from build123d import *

# Parameters (mm, degrees)
SKETCH2_W     = 6.985
SKETCH2_H     = 32.356336156
SKETCH2_W_2   = 40.972237954
SKETCH2_H_2   = 0.889
CUTOUT_DEPTH  = 10.16
TAB_DEPTH     = 2.54
TAB_CHMF_SIZE = 1.524
CROSS_DEPTH   = 7.62
SKETCH4_W     = 3.302
SKETCH4_H     = 7.6962
BOX_DEPTH     = 13.059399
SKETCH6_W     = 1.778
SKETCH6_H     = 6.1722
BOXCUT_DEPTH  = 13.059399
FILLET1_R     = 1.27


with BuildPart() as part:
    # Sketch1 → dome/base (revolve)
    with BuildSketch(Plane.XY):
        with BuildLine():
            Line((0, 6.039891065), (0, 3.960890157))
            Line((0, 3.960890157), (8.222, 3.960890157))
            Line((8.222, 3.960890157), (8.222, -9.047708935))
            Line((8.222, -9.047708935), (10, -9.047708935))
            Line((10, -9.047708935), (10, 4.421422334))
            ThreePointArc((10, 4.421422334), (9.66312833, 5.282916106), (8.831225953, 5.687381775))
            ThreePointArc((8.831225953, 5.687381775), (4.419129287, 5.951728667), (0, 6.039891065))
        make_face()
    revolve(axis=Axis((0, 0, 0), (0, 1, 0)))

    # Sketch2 → cutout (cut)
    with BuildSketch(Plane.XZ.offset(9.047708935)):
        Rectangle(SKETCH2_W, SKETCH2_H)
        with Locations((0, 2.54)):
            Rectangle(SKETCH2_W_2, SKETCH2_H_2)
        with Locations((0, -2.54)):
            Rectangle(SKETCH2_W_2, SKETCH2_H_2)
    extrude(amount=-CUTOUT_DEPTH, mode=Mode.SUBTRACT)

    # Sketch3 → tab (add)
    with BuildSketch(Plane.XZ.offset(9.047708935)):
        with BuildLine():
            Line((-13.169324385, -2.0955), (-9.777979329, -2.0955))
            ThreePointArc((-9.777979329, -2.0955), (-10, 0), (-9.777979329, 2.0955))
            Line((-9.777979329, 2.0955), (-13.169324385, 2.0955))
            ThreePointArc((-13.169324385, 2.0955), (-13.335, 0), (-13.169324385, -2.0955))
        make_face()
        with BuildLine():
            Line((9.777979329, -2.0955), (13.169324385, -2.0955))
            ThreePointArc((13.169324385, -2.0955), (13.293516571, -1.051019583), (13.335, 0))
            ThreePointArc((13.335, 0), (13.293516571, 1.051019583), (13.169324385, 2.0955))
            Line((13.169324385, 2.0955), (9.777979329, 2.0955))
            ThreePointArc((9.777979329, 2.0955), (10, 0), (9.777979329, -2.0955))
        make_face()
    extrude(amount=-TAB_DEPTH)

    # tab chmf
    tab_chmf_edges = [part.edges().sort_by_distance(p)[0] for p in [
        (-13.335, -9.047708935, 0),
        (13.335, -9.047708935, 0),
    ]]
    chamfer(tab_chmf_edges, length=TAB_CHMF_SIZE)

    # Sketch5 → cross (add)
    with BuildSketch(Plane.XZ.offset(-3.960890157)):
        with BuildLine():
            Line((0, -0.71842049), (-0.71842049, 0))
            Line((-0.71842049, 0), (-6.161934605, -5.443514115))
            ThreePointArc((-6.161934605, -5.443514115), (-5.813831955, -5.813831955), (-5.443514115, -6.161934605))
            Line((-5.443514115, -6.161934605), (0, -0.71842049))
        make_face()
        with BuildLine():
            Line((6.161934605, -5.443514115), (0.71842049, 0))
            Line((0.71842049, 0), (0, -0.71842049))
            Line((0, -0.71842049), (5.443514115, -6.161934605))
            ThreePointArc((5.443514115, -6.161934605), (5.813831955, -5.813831955), (6.161934605, -5.443514115))
        make_face()
        with BuildLine():
            Line((5.443514115, 6.161934605), (0, 0.71842049))
            Line((0, 0.71842049), (0.71842049, 0))
            Line((0.71842049, 0), (6.161934605, 5.443514115))
            ThreePointArc((6.161934605, 5.443514115), (5.813831955, 5.813831955), (5.443514115, 6.161934605))
        make_face()
        Polygon((0.71842049, 0), (0, 0.71842049), (-0.71842049, 0), (0, -0.71842049), align=None)
        with BuildLine():
            Line((-0.71842049, 0), (0, 0.71842049))
            Line((0, 0.71842049), (-5.443514115, 6.161934605))
            ThreePointArc((-5.443514115, 6.161934605), (-5.813831955, 5.813831955), (-6.161934605, 5.443514115))
            Line((-6.161934605, 5.443514115), (-0.71842049, 0))
        make_face()
    extrude(amount=CROSS_DEPTH)

    # Sketch4 → box (add)
    with BuildSketch(Plane.XZ.offset(-3.960890157)):
        Rectangle(SKETCH4_W, SKETCH4_H)
    extrude(amount=BOX_DEPTH)

    # Sketch6 → boxcut (cut)
    with BuildSketch(Plane.XZ.offset(9.098508935)):
        Rectangle(SKETCH6_W, SKETCH6_H)
    extrude(amount=-BOXCUT_DEPTH, mode=Mode.SUBTRACT)

    # Fillet1
    fillet1_edges = [part.edges().sort_by_distance(p)[0] for p in [
        (-3.4925, -9.047708935, -8.406831929),
        (3.4925, -9.047708935, -8.406831929),
        (8.602728257, -9.047708935, -2.9845),
        (-8.602728257, -9.047708935, -2.9845),
        (-3.4925, -9.047708935, 8.406831929),
        (3.4925, -9.047708935, 8.406831929),
        (-8.602728257, -9.047708935, 2.9845),
        (8.602728257, -9.047708935, 2.9845),
    ]]
    fillet(fillet1_edges, radius=FILLET1_R)


solid = part.part
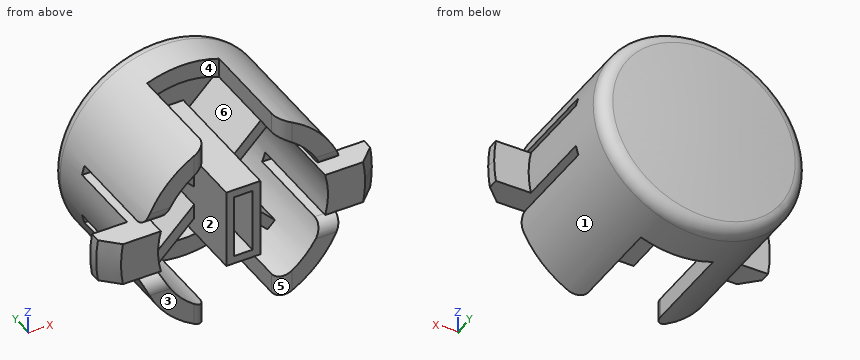
Design review of the part built by this model. Coordinates are the model's own, in mm. Face numbers are marked on the shaded views. A direction names the side the tool comes from. Round coordinates to 2 decimals unless told otherwise and drop trailing zeros. Loops run counter-clockwise (first coordinate to the right, second up) from the corner with the lowest first, then second, coordinate; pieces in that order, holes last. Notation, with made-up numbers: (20.25, 55) - (53.25, 55) arc R14 ccw to (53.25, 81) - close; hole circle Ø4 at (-3, 17.5). An arc over 180 degrees is marked (long way). One line per question, with ' | ' between items.
1. We need section C-C, the plane y = 5. State the section outline as (x, z) points.
Results are:
outline: circle Ø19.72 at (0, 0)
2. We need section B-B, the plane x = 0. State the section outline as (y, z) points.
Results are:
outline: (-9.1, -3.85) - (3.96, -3.85) - (3.96, -8.22) - (1.11, -8.22) - (1.11, -10) - (4.42, -10) arc R1.27 ccw to (5.69, -8.83) arc R110.8 ccw to (5.69, 8.83) arc R1.27 ccw to (4.42, 10) - (1.11, 10) - (1.11, 8.22) - (3.96, 8.22) - (3.96, 3.85) - (-9.1, 3.85) - (-9.1, 3.09) - (3.96, 3.09) - (3.96, -3.09) - (-9.1, -3.09) - close
3. We need section A-A, the plane y = 3. State the section outline as (x, z) points.
Results are:
outline: circle Ø20 at (0, 0); hole (-6.16, -5.44) - (-1.65, -0.93) - (-1.65, 0.93) - (-6.16, 5.44) arc R8.22 ccw to start; hole (-5.44, -6.16) arc R8.22 ccw to (5.44, -6.16) - (1.65, -2.37) - (1.65, -3.85) - (-1.65, -3.85) - (-1.65, -2.37) - close; hole (-5.44, 6.16) - (-1.65, 2.37) - (-1.65, 3.85) - (1.65, 3.85) - (1.65, 2.37) - (5.44, 6.16) arc R8.22 ccw to start; hole (-0.89, -3.09) - (0.89, -3.09) - (0.89, 3.09) - (-0.89, 3.09) - close; hole (1.65, -0.93) - (6.16, -5.44) arc R8.22 ccw to (6.16, 5.44) - (1.65, 0.93) - close
4. Clearance check with flat-ended pins moving along their axes: P1, Ø2, axis at y = -1, z = -4.5, coming from the +X side; P2, Ø1.9, axis at x = 10.5, z = 0.5, coming from the -Y side; P3, Ø3.5, axis at x = 4, z = -2.5, coming from the -Y side. State where each tip first meets the part, or that it passes through.
Results are:
P1: stops at x = 9.37 | P2: stops at y = -9.05 | P3: stops at y = -3.66
5. For the marked faces 4, 5 and 6, list the 3-axis set-ups (+Z, -Z, +X, -X, +Y, -Y) from which the entire face can be reached by the end or side of a thin tool; tool diameter is ignored.
Results are:
face 4: +Z, -Y | face 5: +Z, -Z, -Y | face 6: -Y
6. For L1, parallel to X at y = -2, z = 0; L2, parallel to X at y = -8.5, z = -3.5; L3, parallel to Z at x = 0, y = -4, list the stretches that pass through material, from the lowest coordinate up. Write a range as [from, to].
Results are:
L1: x = [-10, -8.22], [-1.65, -0.89], [0.89, 1.65], [8.22, 10] | L2: x = [-9.37, -7.44], [-1.65, 1.65], [7.44, 9.37] | L3: z = [-3.85, -3.09], [3.09, 3.85]
7. Draft analysis for pull direction Z (two halves, no side actions). For the marked faces 1, 2 and 3, state which applies: released by +Z, released by -Z, zero draft, split by the parting line, or undercut.
Results are:
face 1: split by the parting line | face 2: undercut | face 3: zero draft
